Can you work these out from the model? Positions are in its coordinate system, mm. A direction names the side the tool comes from. Give positions to 0.01 mm unless a question says otherwise; leave off trailing zeros. Loops run counter-clockwise (first coordinate to the right, second up) from the corner with the lowest first, then second, coordinate; pieces in that order, holes last. Notation, with made-up numbers: (78, 4) - (82, 4) arc R9 cw to (82, 16) - close; hole circle Ø7 at (72, 33.25). An arc over 180 degrees is marked (long way). Use a Markdown table: item, result. Add a question column.
Autodesk Inventor part; units mm, degrees
ref_plane "Arbeitsebene1" through (-52.5, 38.3, 0) normal (0, 1, 0) x (1, 0, 0)
ref_plane "Arbeitsebene2" through (-52.5, 40.7, 0) normal (0, 1, 0) x (1, 0, 0)
ref_plane "YZ Plane" through (0, 0, 0) normal (1, 0, 0) x (0, 1, 0)
sketch "Skizze1" plane through (0, 0, 0) normal (0, 0, 1) x (1, 0, 0)
  line L0 (-52.5, 39) -> (52.5, 39)
  line L1 (-52.5, -39) -> (52.5, -39)
  line L2 (52.5, -39) -> (52.5, -43.25)
  line L3 (-52.5, -39) -> (-52.5, -43.25)
  line L4 (-60.5, -43.25) -> (-60.5, 43.25)
  line L5 (-52.5, 39) -> (-52.5, 43.25)
  line L6 (52.5, 39) -> (52.5, 43.25)
  line L7 (60.5, 43.25) -> (60.5, -43.25)
  arc A0 (-52.5, 43.25) -> (-60.5, 43.25) centre (-56.5, 43.25) ccw
  arc A1 (60.5, 43.25) -> (52.5, 43.25) centre (56.5, 43.25) ccw
  arc A2 (52.5, -43.25) -> (60.5, -43.25) centre (56.5, -43.25) ccw
  arc A3 (-60.5, -43.25) -> (-52.5, -43.25) centre (-56.5, -43.25) ccw
  line L8 (0, 66.15) -> (0, -66.15) construction
  line L9 (-84.7, 0) -> (84.7, 0) construction
  circle A4 centre (-56.5, 43.25) radius 1.6
  circle A5 centre (56.5, 43.25) radius 1.6
  circle A6 centre (56.5, -43.25) radius 1.6
  circle A7 centre (-56.5, -43.25) radius 1.6
  point P0 (0, 0)
  dimension "d0" = 121
  dimension "d1" = 78
  dimension "d2" = 8
  dimension "d3" = 86.5
  dimension "d4" = 3.2
extrude "Extrusion1" add sketch "Skizze1" along normal blind 1.6
sketch "Skizze2" plane through (0, 0, 1.6) normal (0, 0, 1) x (1, 0, 0)
  line L0 (-60.5, -38) -> (60.5, -38)
  line L1 (60.5, -38) -> (60.5, 38)
  line L2 (60.5, 38) -> (-60.5, 38)
  line L3 (-60.5, 38) -> (-60.5, -38)
  line L4 (-60.5, -38) -> (60.5, 38) construction
  line L5 (60.5, -38) -> (-60.5, 38) construction
  point P0 (0, 0)
  dimension "d7" = 76
  dimension "d8" = 121
extrude "Extrusion2" add sketch "Skizze2" along normal blind 6.2
ref_plane "Arbeitsebene1" through (-52.5, 38.3, 0) normal (0, 1, 0) x (1, 0, 0)
sketch "Skizze3" plane through (-52.5, 38.3, 0) normal (0, 1, 0) x (1, 0, 0)
  line L0 (60.5, 2.5) -> (60.5, 1)
  line L1 (60.5, 1) -> (61.5, 0)
  line L2 (61.5, 0) -> (67, 0)
  line L3 (67, 0) -> (68, 1)
  line L4 (68, 1) -> (68, 2.5)
  line L5 (68, 2.5) -> (60.5, 2.5)
  line L6 (64.25, 2.5) -> (64.25, 0) construction
  line L7 (79.2, 2.5) -> (79.2, 1)
  line L8 (79.2, 1) -> (80.2, 0)
  line L9 (80.2, 0) -> (85.7, 0)
  line L10 (85.7, 0) -> (86.7, 1)
  line L11 (86.7, 1) -> (86.7, 2.5)
  line L12 (86.7, 2.5) -> (79.2, 2.5)
  line L13 (82.95, 2.5) -> (82.95, 0) construction
  line L14 (0, 0) -> (-8, 0) construction
  line L15 (105, 0) -> (0, 0) construction
  line L16 (113, 0) -> (105, 0) construction
  line L17 (105, 0) -> (113, 0) construction
  line L18 (0, 0) -> (105, 0) construction
  line L19 (-8, 0) -> (0, 0) construction
  line L20 (-2.4, 0) -> (-5.6, 0) construction
  line L21 (110.6, 0) -> (107.4, 0) construction
  line L22 (110.6, 0) -> (107.4, 0) construction
  line L23 (-2.4, 0) -> (-5.6, 0) construction
  line L24 (105, 0) -> (105, -1.6) construction
  line L25 (105, 0) -> (105, -1.6) construction
  point P0 (52.5, 0)
  dimension "d12" = 7.5
  dimension "d13" = 2.5
  dimension "d14" = 1.5
  dimension "d15" = 7.5
  dimension "d16" = 2.5
  dimension "d17" = 1.5
  dimension "d18" = 18.3
  dimension "d19" = 11.2
extrude "Extrusion3" add sketch "Skizze3" against normal blind 5.2
ref_plane "Arbeitsebene2" through (-52.5, 40.7, 0) normal (0, 1, 0) x (1, 0, 0)
sketch "Skizze4" plane through (-52.5, 40.7, 0) normal (0, 1, 0) x (1, 0, 0)
  line L0 (80.2, 0) -> (85.7, 0)
  line L1 (85.7, 0) -> (80.2, 0)
  line L2 (61.5, 0) -> (67, 0)
  line L3 (67, 0) -> (61.5, 0)
  line L4 (0, 0) -> (-8, 0)
  line L5 (105, 0) -> (0, 0)
  line L6 (113, 0) -> (105, 0)
  line L7 (105, 0) -> (113, 0)
  line L8 (0, 0) -> (105, 0)
  line L9 (-8, 0) -> (0, 0)
  line L10 (-2.4, 0) -> (-5.6, 0)
  line L11 (110.6, 0) -> (107.4, 0)
  line L12 (110.6, 0) -> (107.4, 0)
  line L13 (-2.4, 0) -> (-5.6, 0)
  line L14 (105, 0) -> (105, -1.6)
  line L15 (105, 0) -> (105, -1.6)
  line L16 (38.2, 6.4) -> (53.2, 6.4)
  line L17 (53.2, 6.4) -> (53.2, 2.4)
  line L18 (53.2, 2.4) -> (50.8, 0)
  line L19 (50.8, 0) -> (40.6, 0)
  line L20 (40.6, 0) -> (38.2, 2.4)
  line L21 (38.2, 2.4) -> (38.2, 6.4)
  line L22 (45.7, 6.4) -> (45.7, 0) construction
  point P0 (52.5, 0)
  point P1 (40.6, 0)
  point P2 (50.8, 0)
  dimension "d23" = 15
  dimension "d24" = 6.4
  dimension "d25" = 4
  dimension "d26" = 51.8
extrude "Extrusion4" add sketch "Skizze4" against normal blind 12.2
sketch "Skizze5" plane through (-52.5, 39, 1.6) normal (0, 1, 0) x (1, 0, 0)
  line L0 (20.7, 6.6) -> (26.7, 6.6)
  line L1 (26.7, 6.6) -> (26.7, 1.6)
  line L2 (26.7, 1.6) -> (20.7, 1.6)
  line L3 (20.7, 1.6) -> (20.7, 6.6)
  line L4 (105, 1.6) -> (50.8, 1.6)
  line L5 (113, 1.6) -> (105, 1.6)
  line L6 (105, 1.6) -> (113, 1.6)
  line L7 (0, 1.6) -> (105, 1.6)
  line L8 (-8, 1.6) -> (0, 1.6)
  line L9 (0, 1.6) -> (-8, 1.6)
  line L10 (40.6, 1.6) -> (0, 1.6)
  line L11 (40.6, 1.6) -> (50.8, 1.6)
  line L12 (80.2, 1.6) -> (85.7, 1.6)
  line L13 (85.7, 1.6) -> (80.2, 1.6)
  line L14 (61.5, 1.6) -> (67, 1.6)
  line L15 (67, 1.6) -> (61.5, 1.6)
  line L16 (-2.4, 1.6) -> (-5.6, 1.6)
  line L17 (110.6, 1.6) -> (107.4, 1.6)
  line L18 (110.6, 1.6) -> (107.4, 1.6)
  line L19 (-2.4, 1.6) -> (-5.6, 1.6)
  line L20 (40.6, 1.6) -> (0, 1.6)
  line L21 (105, 1.6) -> (105, 0)
  point P0 (52.5, 1.6)
  dimension "d29" = 5
  dimension "d30" = 6
  dimension "d31" = 78.3
extrude "Extrusion5" add sketch "Skizze5" against normal blind 12.2
sketch "Skizze6" plane through (-52.5, 39, 1.6) normal (0, 1, 0) x (1, 0, 0)
  line L0 (26.7, 6.6) -> (20.7, 6.6)
  line L1 (20.7, 6.6) -> (20.7, 1.6)
  line L2 (26.7, 1.6) -> (26.7, 6.6)
  line L3 (20.7, 6.6) -> (26.7, 1.6) construction
  line L4 (26.7, 6.6) -> (20.7, 1.6) construction
  circle A0 centre (23.7, 4.1) radius 2.5
  circle A1 centre (23.7, 4.1) radius 1.5
  point P0 (52.5, 1.6)
  dimension "d34" = 3
extrude "Extrusion6" add sketch "Skizze6" along normal blind 1.8
sketch "Skizze7" plane through (0, 0, 0) normal (0, 0, -1) x (-1, 0, 0)
  line L0 (-42.3, 35.2) -> (-47.1, 35.2)
  line L1 (-47.1, 35.2) -> (-47.1, 38.8)
  line L2 (-42.3, 38.8) -> (-42.3, 35.2)
  line L3 (-46, 38.8) -> (-46, 40)
  line L4 (-46, 40) -> (-43.4, 40)
  line L5 (-43.4, 40) -> (-43.4, 38.8)
  line L6 (-47.1, 38.8) -> (-46, 38.8)
  line L7 (-43.4, 38.8) -> (-42.3, 38.8)
  line L8 (-44.7, 35.2) -> (-44.7, 40) construction
  line L9 (-52.5, 43.25) -> (-52.5, 39) construction
  line L10 (-52.5, 39) -> (1.7, 39) construction
  point P0 (0, 0)
  dimension "d37" = 2.6
  dimension "d38" = 1.2
  dimension "d39" = 3.6
  dimension "d40" = 4.8
  dimension "d41" = 5.4
  dimension "d42" = 1
extrude "Extrusion7" add sketch "Skizze7" along normal blind 1.8
properties part number "Display 5inch JRP5002"
1. Please list where these lines run through material, in increasing order: line 1 along Y through (x, z) = (56.5, 1); line 2 along Z through (x, y) = (-28.8, 39.85); line 3 along Z through (x, y) = (26, -22.5). Write a range as [from, to].
2. Suppose I cut it at B-B (x = -34). List the corners of the cut face in (y, z) for me.
3. Suppose I cut it at D-D (y = -4). List the corners of the cut face in (x, z) for me.
4. If we mould it in two halves opening along Y, with no side actions, what happens to faces 4 (the face through (57.98, -42.64, 0.79)), 5 (the face through (-7, 28.5, -3)), 6 (the face through (1, 38, 5)), 7 (the face through (-14.3, 35, -4))? For each: released by +Y, released by -Y, zero draft, split by the parting line, or undercut.
5. On a 3-axis mill with a long thin cutter (end or side, diameter ignored), from which of +Z, -Z, +X, -X, +Y, -Y can I reach the whole of each face in a straight line? I mean faces 1 (the face through (12, 38.3, -1)), 2 (the face through (-1, -38, 5)), 3 (the face through (-31.8, 33, -2)). Say none if no direction works.
6. Will these pins go through, and if not, where does the flat tip stop? P1, Ø1, axis at x = 14.5, y = 4.5, coming from the -Z side; P2, Ø1.5, axis at x = -27.5, z = -3, coming from the +Y side; P3, Ø4, axis at x = 31, y = 34.5, coming from the -Z side; P4, Ø3, axis at x = 56.5, y = -43.25, coming from the +Z side.
7. Suppose I cut it at A-A (x = -56.5). List the corners of the cut face in (y, z) for me.
8. Suppose I cut it at C-C (z = 4.5). List the corners of the cut face in (x, y) for me.
Results below:
| question | item | result |
|---|---|---|
| 1 | line 1 | [-47.25, -44.85], [-41.65, 41.65], [44.85, 47.25] |
| 1 | line 2 | [-5, -4], [-1, 0] |
| 1 | line 3 | [0, 7.8] |
| 2 | outline | (-39, 0) - (39, 0) - (39, 1.6) - (38, 1.6) - (38, 7.8) - (-38, 7.8) - (-38, 1.6) - (-39, 1.6) - close |
| 3 | outline | (-60.5, 0) - (60.5, 0) - (60.5, 7.8) - (-60.5, 7.8) - close |
| 4 | face 4 | undercut |
| 4 | face 5 | released by -Y |
| 4 | face 6 | released by +Y |
| 4 | face 7 | zero draft |
| 5 | face 1 | -Z, +Y |
| 5 | face 2 | +Z, +X, -X, -Y |
| 5 | face 3 | -Z, -X, +Y, -Y |
| 6 | P1 | z = 0 |
| 6 | P2 | y = 40.8 |
| 6 | P3 | z = -2.5 |
| 6 | P4 | through |
| 7 | outline | (-47.25, 0) - (-44.85, 0) - (-44.85, 1.6) - (-47.25, 1.6) - close; (-41.65, 0) - (41.65, 0) - (41.65, 1.6) - (38, 1.6) - (38, 7.8) - (-38, 7.8) - (-38, 1.6) - (-41.65, 1.6) - close; (44.85, 0) - (47.25, 0) - (47.25, 1.6) - (44.85, 1.6) - close |
| 8 | outline | (-60.5, -38) - (60.5, -38) - (60.5, 38) - (-60.5, 38) - close |
